Read the model definition and answer for the solid it produces. Units are mm, in the model's axes. Coordinates: 2 decimals unless noted, no trailing zeros. Order: outer loops, then holes, each group sorted by start corner. A loop starts at its lowest first (then second) coordinate and runs counter-clockwise, first axis right, second up. Notation, with made-up numbers: M 87,-14.5 L 103,-14.5 A29 ccw 103,12.5 Z; hole C -22,-16 d1. An arc over 180 degrees is marked long. Use a Markdown table: item, result. Add a question column.
1) Find the intervals of material crossed by probe 1 along X at (y, z) = (-90, 0.4); probe 2 along X at (y, z) = (0, 0.3); probe 3 along Y at (x, z) = (0, 0.7) (3 decimals), in increasing order. Write a range as [from, to].
2) Find section C-C on x = 44.9. Write down the section's boundary in (y, z).
3) Find section B-B on x = -26. Write down the section's boundary in (y, z), plus the area to 3 significant figures.
4) Find section A-A on y = 90. Write down the section's boundary in (x, z).
Solid Edge part; units mm, degrees
sketch "Sketch1" plane through (0, 0, 0) normal (0, 0, 1) x (1, 0, 0)
  line L0 (-52, -100) -> (52, -100)
  line L1 (52, -100) -> (52, 100)
  line L2 (52, 100) -> (-52, 100)
  line L3 (-52, 100) -> (-52, -100)
extrude "Extrusionsausprägung_1" add sketch "Sketch1" along normal blind 0.9
hole "Bohrung_1" at (-44.9, 90, 0.9) direction (0, 0, -1) diameter 6.4 end up to next
hole "Hole1" at (44.9, 90, 0.9) direction (0, 0, -1) diameter 6.4 end up to next
hole "Hole2" at (44.9, -90, 0.9) direction (0, 0, -1) diameter 6.4 end up to next
hole "Hole3" at (-44.9, -90, 0.9) direction (0, 0, -1) diameter 6.4 end up to next
hole "Bohrung_5" at (-26, 0, 0.9) direction (0, 0, -1) diameter 4.3 end up to next
hole "Hole4" at (26, 0, 0.9) direction (0, 0, -1) diameter 4.3 end up to next
hole "Bohrung_7" at (0, 38, 0.9) direction (0, 0, -1) diameter 2.15 end up to next
hole "Hole5" at (0, -38, 0.9) direction (0, 0, -1) diameter 2.15 end up to next
properties material "Aluminium, 2024-T4"
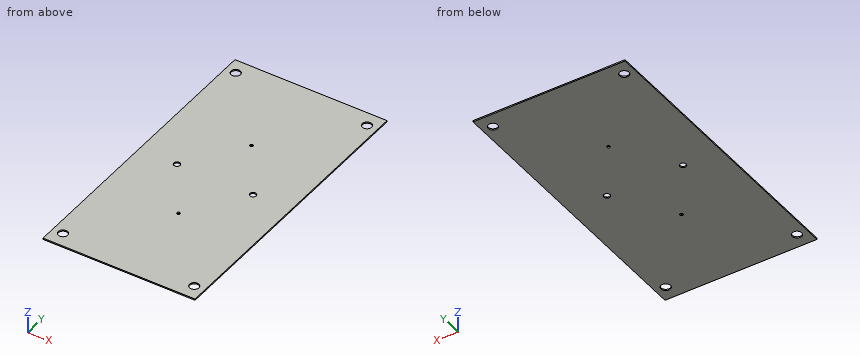
Check result:
| question | item | result |
|---|---|---|
| 1 | probe 1 | x = [-52, -48.1], [-41.7, 41.7], [48.1, 52] |
| 1 | probe 2 | x = [-52, -28.15], [-23.85, 23.85], [28.15, 52] |
| 1 | probe 3 | y = [-100, -39.075], [-36.925, 36.925], [39.075, 100] |
| 2 | outline | M -100,0 L -93.2,0 L -93.2,0.9 L -100,0.9 Z; M -86.8,0 L 86.8,0 L 86.8,0.9 L -86.8,0.9 Z; M 93.2,0 L 100,0 L 100,0.9 L 93.2,0.9 Z |
| 3 | outline | M -100,0 L -2.15,0 L -2.15,0.9 L -100,0.9 Z; M 2.15,0 L 100,0 L 100,0.9 L 2.15,0.9 Z |
| 3 | area | 176 mm2 |
| 4 | outline | M -52,0 L -48.1,0 L -48.1,0.9 L -52,0.9 Z; M -41.7,0 L 41.7,0 L 41.7,0.9 L -41.7,0.9 Z; M 48.1,0 L 52,0 L 52,0.9 L 48.1,0.9 Z |
